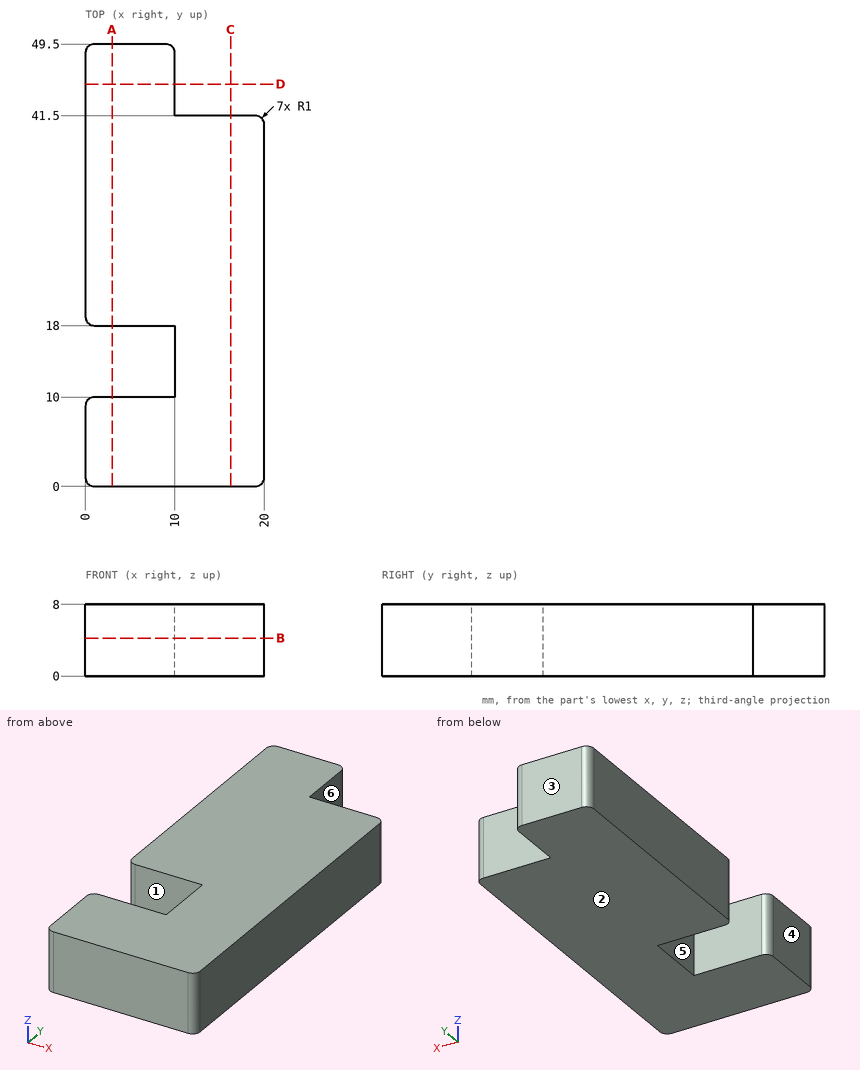
Here's the drawing with two shaded views (mm, measured from the low corner). I have some questions. A direction names the side the tool comes from. Round coordinates to 2 decimals unless told otherwise and drop trailing zeros. Loops run counter-clockwise (first coordinate to the right, second up) from the corner with the lowest first, then second, coordinate; pieces in that order, holes last. Notation, with made-up numbers: M 87,-30 L 122,-30 A7 ccw 122,-20 Z; hole C 42,77.25 d7. An arc over 180 degrees is marked long. Answer as a JSON object with one key per item and string values. Group by question number.
Q1. Will these pins go through, and if not, where does the flat tip stop? pin 1 (2.5 mm diameter, centred on x = 16.5, z = 5, fed in from +Y); pin 2 (3.5 mm diameter, centred on y = 45, z = 5, fed in from +X).
Q2. Imagine slicing it at B-B, the plane z = 4.25. Please give me the cut outline in (x, y), then the cut area to 4 significant figures.
Q3. Please list where these lines run through material, in increasing order: L1, parallel to Y at x = 8.5, z = 1.75; L2, parallel to Y at x = 10.5, z = 1.5; L3, parallel to X at y = 44.5, z = 6.25.
Q4. Imagine slicing it at C-C, the plane x = 16.25. Please give me the cut outline in (y, z).
Q5. Imagine slicing it at D-D, the plane y = 45. Please give me the cut outline in (x, z), then the cut area to 3 significant figures.
Q6. On a 3-axis mill with a long thin cutter (end or side, diameter ignored), from which of +Z, -Z, +X, -X, +Y, -Y can I reach the whole of each face in a straight line? I mean the marked faces 4, 5 and 6. Say none if no direction works.
Q7. Imagine slicing it at A-A, the plane x = 3. Please give me the cut outline in (y, z), then the cut area to 3 significant figures.
Q8. We'd pull the mould along Y, two halves only. Please class the marked faces 1, 2 and 3: +Y half, -Y half, draft (parallel to the pull), parting line (faces both ways), or undercut.
Findings:
{
 "1": {"pin 1": "stops at y = 41.5", "pin 2": "stops at x = 10"},
 "2": {"outline": "M 0,1 A1 ccw 1,0 L 19,0 A1 ccw 20,1 L 20,40.5 A1 ccw 19,41.5 L 10,41.5 L 10,48.5 A1 ccw 9,49.5 L 1,49.5 A1 ccw 0,48.5 L 0,19 A1 ccw 1,18 L 10,18 L 10,10 L 1,10 A1 ccw 0,9 Z", "area": "828.5 mm2"},
 "3": {"L1": "y = 0 to 10, 18 to 49.5", "L2": "y = 0 to 41.5", "L3": "x = 0 to 10"},
 "4": {"outline": "M 0,0 L 41.5,0 L 41.5,8 L 0,8 Z"},
 "5": {"outline": "M 0,0 L 10,0 L 10,8 L 0,8 Z", "area": "80.0 mm2"},
 "6": {"face 4": "+Z, -Z, -X, +Y, -Y", "face 5": "+Z, -Z, -X", "face 6": "+Z, -Z, +X, +Y"},
 "7": {"outline": "M 0,0 L 10,0 L 10,8 L 0,8 Z; M 18,0 L 49.5,0 L 49.5,8 L 18,8 Z", "area": "332 mm2"},
 "8": {"face 1": "undercut", "face 2": "draft", "face 3": "+Y half"}
}
